```python
from build123d import *

# Parameters (mm, degrees)
F1_DEPTH = 6.35
F2_R     = 5.08


with BuildPart() as f1:
    # F0 (on Front) → F1 (new body)
    with BuildSketch(Plane.XZ):
        with BuildLine():
            Line((74.237378, 112.354313), (-119.437622, 112.354313))
            Line((-119.437622, 112.354313), (-119.437622, -90.845687))
            Line((-119.437622, -90.845687), (-94.037622, -90.845687))
            Line((-94.037622, -90.845687), (-94.037622, 52.75996))
            ThreePointArc((-94.037622, 52.75996), (-81.337622, 65.45996), (-68.637622, 52.75996))
            Line((-68.637622, 52.75996), (-68.637622, -90.845687))
            Line((-68.637622, -90.845687), (-43.237622, -90.845687))
            Line((-43.237622, -90.845687), (-43.237622, 52.771378))
            ThreePointArc((-43.237622, 52.771378), (-30.537622, 65.471378), (-17.837622, 52.771378))
            Line((-17.837622, 52.771378), (-17.837622, -90.845687))
            Line((-17.837622, -90.845687), (23.437378, -90.845687))
            Line((23.437378, -90.845687), (23.437378, 51.066604))
            ThreePointArc((23.437378, 51.066604), (36.137378, 63.766604), (48.837378, 51.066604))
            Line((48.837378, 51.066604), (48.837378, -90.845687))
            Line((48.837378, -90.845687), (74.237378, -90.845687))
            Line((74.237378, -90.845687), (74.237378, 112.354313))
        make_face()
    extrude(amount=-F1_DEPTH)

    # F2
    f2_edges = [f1.edges().sort_by_distance(p)[0] for p in [
        (-94.037622, 3.175, -90.845687),
        (-68.637622, 3.175, -90.845687),
        (-43.237622, 3.175, -90.845687),
        (-17.837622, 3.175, -90.845687),
        (23.437378, 3.175, -90.845687),
        (48.837378, 3.175, -90.845687),
        (74.237378, 3.175, -90.845687),
        (-119.437622, 3.175, -90.845687),
    ]]
    fillet(f2_edges, radius=F2_R)


solid = f1.part
```
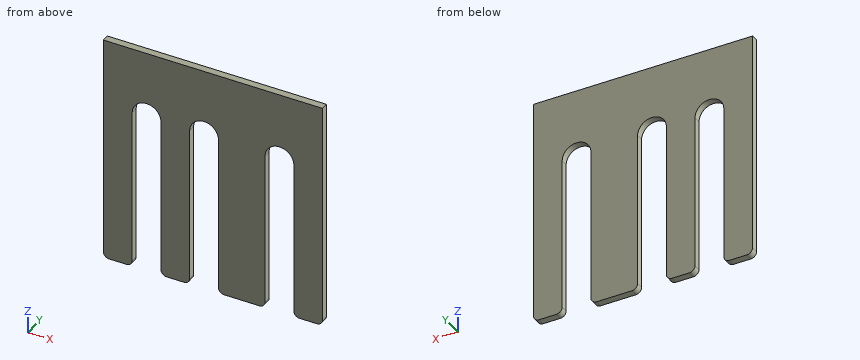
Build history of the part. All positions in model axes, mm. Round coordinates to 2 decimals unless told otherwise and drop trailing zeros. Order: outer loops, then holes, each group sorted by start corner. A loop starts at its lowest first (then second) coordinate and runs counter-clockwise, first axis right, second up. Notation, with made-up numbers: (-26.5, 27) -> (-0.5, 27) arc R8 cw to (-0.5, 42) -> close; hole circle Ø2 at (-12, 32.5). An arc over 180 degrees is marked (long way). Answer in a Markdown table with one row per item.
1) Band-saw the part on B-B on y = 1.5. Give the cut face in (x, z), and give its area (3 significant figures).
Values:
| item | result |
|---|---|
| outline | (-119.44, -85.77) arc R5.08 ccw to (-114.36, -90.85) -> (-99.12, -90.85) arc R5.08 ccw to (-94.04, -85.77) -> (-94.04, 52.76) arc R12.7 cw to (-68.64, 52.76) -> (-68.64, -85.77) arc R5.08 ccw to (-63.56, -90.85) -> (-48.32, -90.85) arc R5.08 ccw to (-43.24, -85.77) -> (-43.24, 52.77) arc R12.7 cw to (-17.84, 52.77) -> (-17.84, -85.77) arc R5.08 ccw to (-12.76, -90.85) -> (18.36, -90.85) arc R5.08 ccw to (23.44, -85.77) -> (23.44, 51.07) arc R12.7 cw to (48.84, 51.07) -> (48.84, -85.77) arc R5.08 ccw to (53.92, -90.85) -> (69.16, -90.85) arc R5.08 ccw to (74.24, -85.77) -> (74.24, 112.35) -> (-119.44, 112.35) -> close |
| area | 27,700 mm2 |
2) Band-saw the part on A-A on z = 13.5. Give the cut face in (x, y).
Values:
| item | result |
|---|---|
| outline | (-119.44, 0) -> (-94.04, 0) -> (-94.04, 6.35) -> (-119.44, 6.35) -> close; (-68.64, 0) -> (-43.24, 0) -> (-43.24, 6.35) -> (-68.64, 6.35) -> close; (-17.84, 0) -> (23.44, 0) -> (23.44, 6.35) -> (-17.84, 6.35) -> close; (48.84, 0) -> (74.24, 0) -> (74.24, 6.35) -> (48.84, 6.35) -> close |
3) Wall check: L1, parallel to X at y = 1.25, z = -30; L2, parallel to X at y = 3.25, z = 54.5; L3, parallel to Z at x = -13.5, y = 3.25. Give the ranges that are in metal, low to high.
Values:
| item | result |
|---|---|
| L1 | -119.44 to -94.04, -68.64 to -43.24, -17.84 to 23.44, 48.84 to 74.24 |
| L2 | -119.44 to -93.92, -68.76 to -43.12, -17.96 to 23.91, 48.36 to 74.24 |
| L3 | -90.79 to 112.35 |
4) Band-saw the part on C-C on z = 56.5. Give the cut face in (x, y).
Values:
| item | result |
|---|---|
| outline | (-119.44, 0) -> (-93.47, 0) -> (-93.47, 6.35) -> (-119.44, 6.35) -> close; (-69.2, 0) -> (-42.68, 0) -> (-42.68, 6.35) -> (-69.2, 6.35) -> close; (-18.4, 0) -> (24.66, 0) -> (24.66, 6.35) -> (-18.4, 6.35) -> close; (47.62, 0) -> (74.24, 0) -> (74.24, 6.35) -> (47.62, 6.35) -> close |
5) Band-saw the part on D-D on x = -89. Give the cut face in (y, z).
Values:
| item | result |
|---|---|
| outline | (0, 62.89) -> (6.35, 62.89) -> (6.35, 112.35) -> (0, 112.35) -> close |
